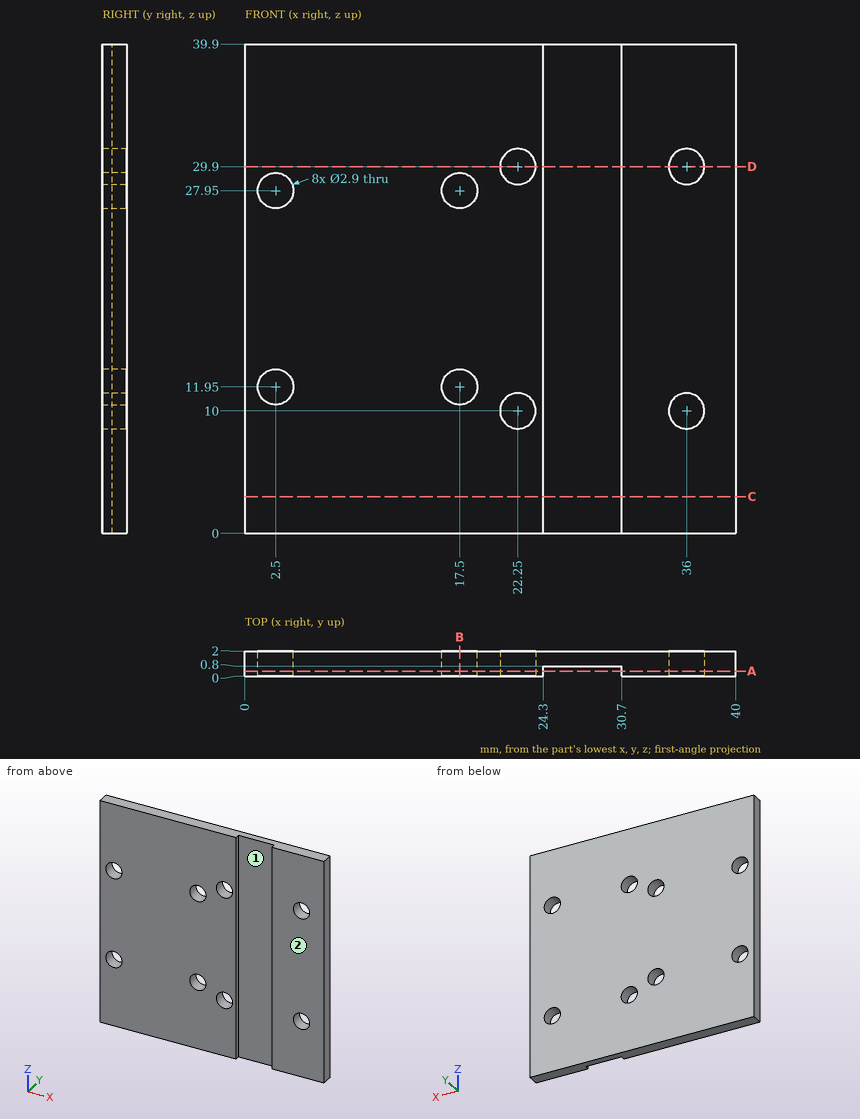
Check sheet for the drawn part. Datum: minimum x, y, z corner. Units: mm. Round coordinates to 2 decimals unless told otherwise and drop trailing zeros. Loops run counter-clockwise (first coordinate to the right, second up) from the corner with the lowest first, then second, coordinate; pieces in that order, holes last. Notation, with made-up numbers: (-6, 64.25) - (43, 64.25) arc R14 ccw to (43, 76.25) - close; hole circle Ø2 at (61.25, -40). An arc over 180 degrees is marked (long way). Answer as a JSON object with one key per item and string values. Group by question number.
Q1. Sectioned sample at C-C, the plane z = 3. Enter the section's corners in (x, y).
Q2. Mould release check, pull along X, two halves, no side actions. Record for the marked faces 1 and 2: released by +X, released by -X, zero draft, split by the parting line, or undercut.
Q3. Sectioned sample at D-D, the plane z = 29.9. Enter the section's corners in (x, y).
Q4. Sectioned sample at A-A, the plane y = 0.4. Count the separate pieces of the cut face and the enclosed holes in it, plus the area to 3 significant figures.
Q5. Sectioned sample at B-B, the plane x = 17.5. Enter the section's corners in (y, z).
Q6. Scan lines: line 1 along X through (y, z) = (1, 27.95); line 2 along X through (y, z) = (1.4, 29.9); line 3 along X through (y, z) = (0.45, 33.5). Record each from-to range of solid material in increasing order. Write a range as [from, to].
Q7. Gauge pin test, flat ends, axial feed: P1, Ø3.5, axis at x = 17.5, z = 11.95, coming from the +Y side; P2, Ø1.9, axis at x = 29, z = 11, coming from the -Y side. Record the tip position at first contact, or that the pin passes through.
Solution:
{
 "1": {"outline": "(0, 0) - (24.3, 0) - (24.3, 0.8) - (30.7, 0.8) - (30.7, 0) - (40, 0) - (40, 2) - (0, 2) - close"},
 "2": {"face 1": "undercut", "face 2": "zero draft"},
 "3": {"outline": "(0, 0) - (20.8, 0) - (20.8, 2) - (0, 2) - close; (23.7, 0) - (24.3, 0) - (24.3, 0.8) - (30.7, 0.8) - (30.7, 0) - (34.55, 0) - (34.55, 2) - (23.7, 2) - close; (37.45, 0) - (40, 0) - (40, 2) - (37.45, 2) - close"},
 "4": {"separate pieces": "2", "enclosed holes": "8", "area": "1,290 mm²"},
 "5": {"outline": "(0, 0) - (2, 0) - (2, 10.5) - (0, 10.5) - close; (0, 13.4) - (2, 13.4) - (2, 26.5) - (0, 26.5) - close; (0, 29.4) - (2, 29.4) - (2, 39.9) - (0, 39.9) - close"},
 "6": {"line 1": "x = [0, 1.05], [3.95, 16.05], [18.95, 40]", "line 2": "x = [0, 20.8], [23.7, 34.55], [37.45, 40]", "line 3": "x = [0, 24.3], [30.7, 40]"},
 "7": {"P1": "stops at y = 2", "P2": "stops at y = 0.8"}
}
